Geometry: see drawing. Coordinates: mm, zero at the bounding-box minimum. Coordinates: 2 decimals unless noted, no trailing zeros. Loops run counter-clockwise (first coordinate to the right, second up) from the corner with the lowest first, then second, coordinate; pieces in that order, holes last.
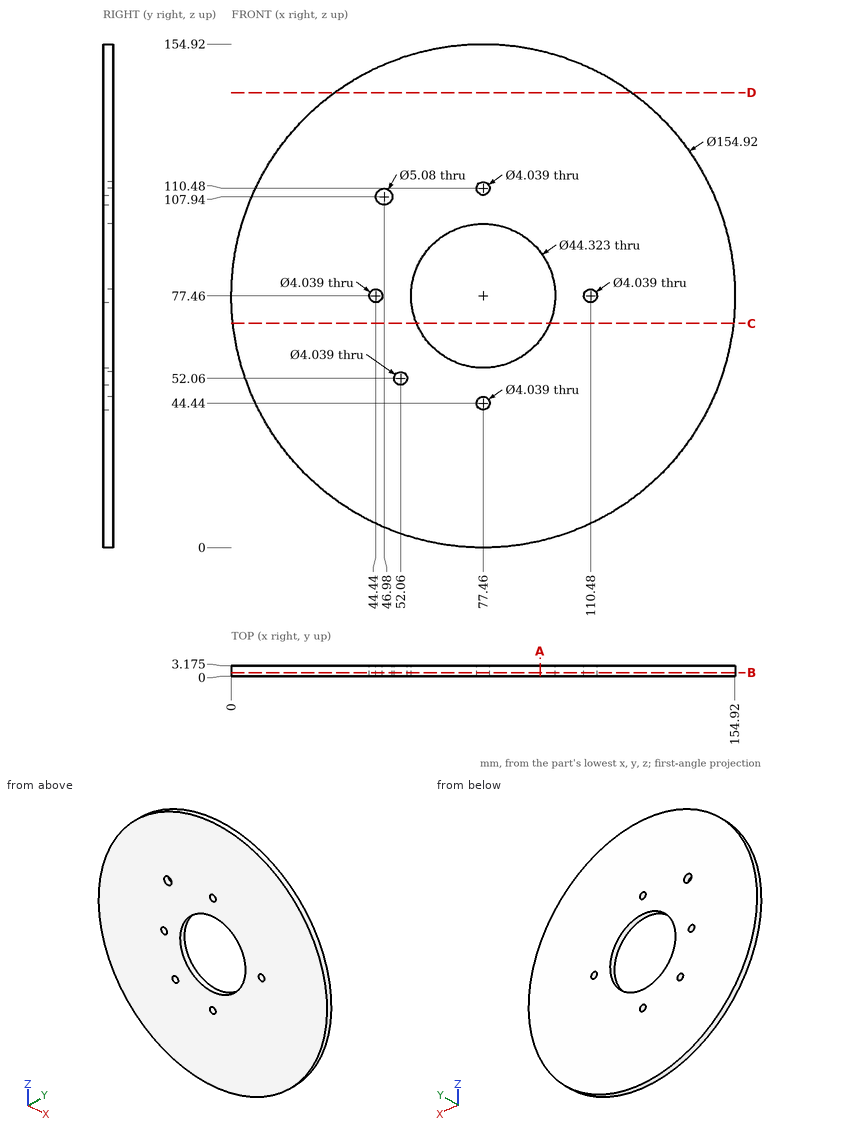
Item 1: Line query: L1, parallel to X at y = 2.3, z = 73; L2, parallel to X at y = 2.15, z = 64.5 (1 decimal); L3, parallel to Z at x = 85.5, y = 1.85. Output: solid intervals per line, ascending.
Result:
L1: x = 0.13 to 55.75, 99.17 to 154.79
L2: x = 1.1 to 59.5, 95.4 to 153.8
L3: z = 0.42 to 56.81, 98.11 to 154.5
Item 2: Section query C-C (z = 69). Output: boundary loops of the cut face in (x, y) (1 decimal), then the cut area to 3 significant figures.
Result:
outline: (0.5, 0) - (57, 0) - (57, 3.2) - (0.5, 3.2) - close; (97.9, 0) - (154.5, 0) - (154.5, 3.2) - (97.9, 3.2) - close
area: 359 mm2
Item 3: Contact query for a flat-ended pin moving along its axis: P1, Ø3, axis at x = 44.44, z = 77.46, coming from the +Y side. Output: stop coordinate, or through.
Result:
P1: passes through
Item 4: Section query B-B (y = 1). Output: boundary loops of the cut face in (x, z), then the cut area to 3 significant figures.
Result:
outline: circle Ø154.92 at (77.46, 77.46); hole circle Ø4.04 at (44.44, 77.46); hole circle Ø5.08 at (46.98, 107.94); hole circle Ø4.04 at (52.06, 52.06); hole circle Ø44.32 at (77.46, 77.46); hole circle Ø4.04 at (77.46, 44.44); hole circle Ø4.04 at (77.46, 110.48); hole circle Ø4.04 at (110.48, 77.46)
area: 17,200 mm2
Item 5: Section query D-D (z = 140). Output: boundary loops of the cut face in (x, y) (1 decimal), then the cut area to 3 significant figures.
Result:
outline: (31.8, 0) - (123.2, 0) - (123.2, 3.2) - (31.8, 3.2) - close
area: 290 mm2
Item 6: Section query A-A (x = 95). Output: boundary loops of the cut face in (y, z) (1 decimal), then the cut area to 3 significant figures.
Result:
outline: (0, 2) - (3.2, 2) - (3.2, 63.9) - (0, 63.9) - close; (0, 91) - (3.2, 91) - (3.2, 152.9) - (0, 152.9) - close
area: 393 mm2
